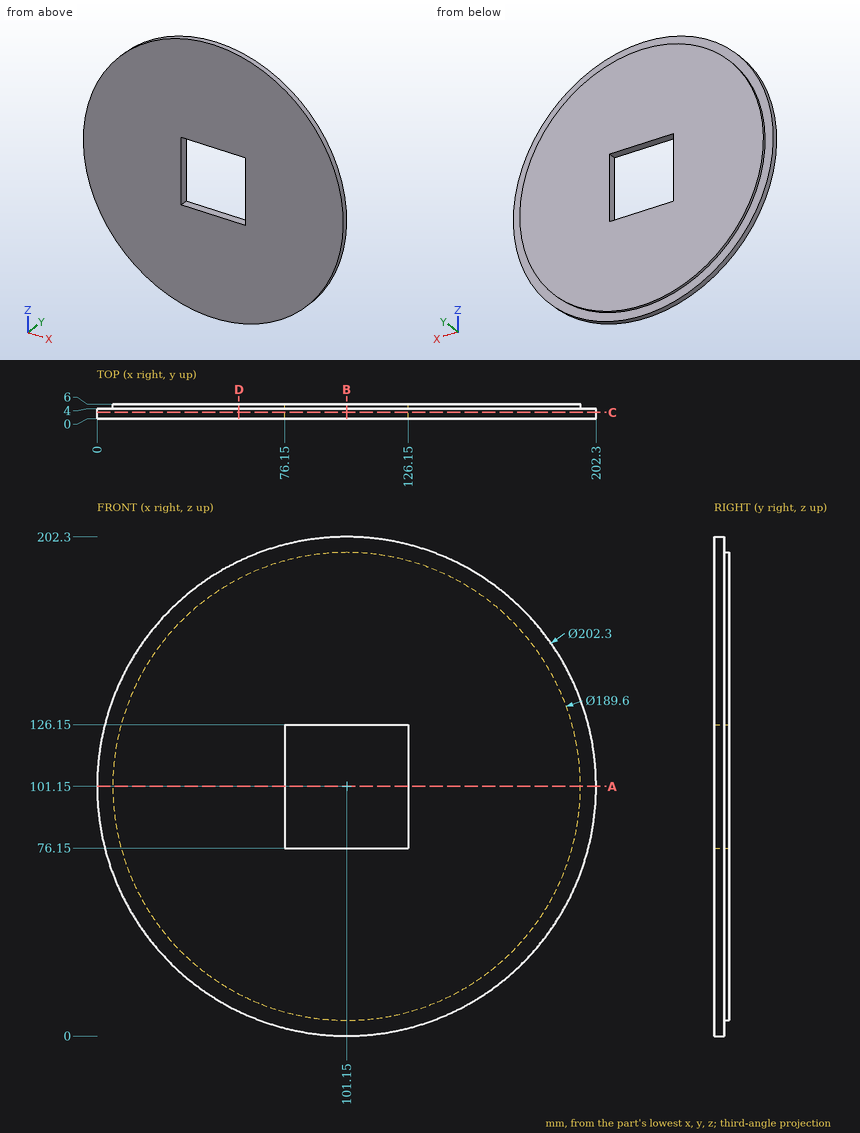
Geometry: see drawing. Coordinates: mm, zero at the bounding-box minimum. Coordinates: 2 decimals unless noted, no trailing zeros. Order: outer loops, then holes, each group sorted by start corner. A loop starts at its lowest first (then second) coordinate and runs counter-clockwise, first axis right, second up. Notation, with made-up numbers: M 19.5,65 L 45.5,65 A8 ccw 45.5,74 Z; hole C -26.75,37.5 d4. An arc over 180 degrees is marked long. Write each question's results on one line, items separated by ' | '. Start each with the question number.
1) Section query B-B (x = 101.15). Return the cut outline in (y, z), plus the area to 3 significant figures.
2) Contact query for flat-ended pins moving along their axis: pin 1 Ø2 at (x, y) = (80.5, 4) entering from -Z; pin 2 Ø1.5 at (x, y) = (47.5, 1.5) entering from -Z; pin 3 Ø1 at (x, z) = (116, 58.5) entering from -Y; pin 4 Ø3 at (y, z) = (4, 98.5) entering from +X. Output: stop coordinate, or through.
3) Line query: line 1 (Z direction, x = 99, y = 2.6); line 2 (Z direction, x = 84, y = 4.8); line 3 (X direction, y = 3.5, z = 112). Output: solid intervals per line, ascending. Write a range as from..to.
4) Section query A-A (z = 101.15). Return the cut outline in (x, y), plus the area to 3 significant figures.
5) Section query C-C (y = 2.65). Return the cut outline in (x, z), plus the area to 3 significant figures.
6) Section query D-D (x = 57.5). Return the cut outline in (y, z).
Answers:
1) outline: M 0,0 L 4,0 L 4,6.35 L 6,6.35 L 6,76.15 L 0,76.15 Z; M 0,126.15 L 6,126.15 L 6,195.95 L 4,195.95 L 4,202.3 L 0,202.3 Z | area: 888 mm^2
2) pin 1: stops at z = 1.93 | pin 2: stops at z = 14.94 | pin 3: stops at y = 0 | pin 4: stops at x = 202.29
3) line 1: z = 0.02..76.15, 126.15..202.28 | line 2: z = 7.91..76.15, 126.15..194.39 | line 3: x = 0.58..76.15, 126.15..201.72
4) outline: M 0,0 L 76.15,0 L 76.15,6 L 6.35,6 L 6.35,4 L 0,4 Z; M 126.15,0 L 202.3,0 L 202.3,4 L 195.95,4 L 195.95,6 L 126.15,6 Z | area: 888 mm^2
5) outline: C 101.15,101.15 d202.3; hole M 76.15,76.15 L 126.15,76.15 L 126.15,126.15 L 76.15,126.15 Z | area: 29,600 mm^2
6) outline: M 0,9.9 L 4,9.9 L 4,17 L 6,17 L 6,185.3 L 4,185.3 L 4,192.4 L 0,192.4 Z
